```python
from build123d import *

# Parameters (mm, degrees)
SKETCH1_W           = 6
SKETCH1_H           = 6
BOSS_EXTRUDE1_DEPTH = 5
CUT_EXTRUDE1_DEPTH  = 1
CUT_EXTRUDE2_DEPTH  = 2
CUT_EXTRUDE3_DEPTH  = 2


with BuildPart() as part:
    # Sketch1 → Boss-Extrude1 (new body)
    with BuildSketch(Plane(origin=(0, 0, 0), x_dir=(1, 0, 0), z_dir=(0, 1, 0))):
        Rectangle(SKETCH1_W, SKETCH1_H)
    extrude(amount=BOSS_EXTRUDE1_DEPTH)

    # Sketch2 → Cut-Extrude1 (cut, symmetric)
    with BuildSketch(Plane(origin=(0, 0, 0), x_dir=(0, 0, -1), z_dir=(1, 0, 0))):
        Polygon((-3, 0), (3, 0), (3, 1), align=None)
        Polygon((3, 5), (-3, 5), (-3, 3), align=None)
    extrude(amount=CUT_EXTRUDE1_DEPTH, both=True, mode=Mode.SUBTRACT)

    # Sketch3 → Cut-Extrude2 (cut)
    with BuildSketch(Plane.ZY.offset(3)):
        Polygon((-3, 4), (3, 2), (3, 5), (-3, 5), align=None)
    extrude(amount=-CUT_EXTRUDE2_DEPTH, mode=Mode.SUBTRACT)

    # Sketch4 → Cut-Extrude3 (cut)
    with BuildSketch(Plane.ZY.offset(-1)):
        Polygon((3, 5), (-3, 5), (3, 4), align=None)
    extrude(amount=-CUT_EXTRUDE3_DEPTH, mode=Mode.SUBTRACT)


solid = part.part
```
The listing builds one solid part. Answer for the finished solid, in the listing's coordinates (mm). A direction names the side the tool comes from. Coordinates: 2 decimals unless noted, no trailing zeros. Loops run counter-clockwise (first coordinate to the right, second up) from the corner with the lowest first, then second, coordinate; pieces in that order, holes last. Notation, with made-up numbers: (62, 31.5) -> (66, 31.5) arc R11 ccw to (66, 39.5) -> close; hole circle Ø10 at (-27.75, 29.25). An arc over 180 degrees is marked (long way). Return JSON: item names as keys, results as strings. Group by question number.
(1) A cutting plane is placed at D-D on y = 2.55. Write down the section's boundary in (x, z), and give its area (3 significant figures).
(2) A cutting plane is placed at C-C on x = 1.85. Write down the section's boundary in (y, z).
(3) A cutting plane is placed at B-B on z = 2. Write down the section's boundary in (x, y).
(4) A cutting plane is placed at A-A on y = 3.55. Write down the section's boundary in (x, z), and give its area (3 significant figures).
(5) Which of the six approach directions +Z, -Z, +X, -X, +Y, -Y give full straight-line access (tool end or side, diameter ignored) to faces 1 (the flat face through (-2, 0, 0)), 2 (the flat face through (-1, 0.3, -1.3)), 3 (the flat face through (-1, 3.6, 0))?
(6) Find the intervals of material crossed by probe 1 along X at (y, z) = (3.65, -1.25); probe 2 along X at (y, z) = (0.55, -1.5); probe 3 along Y at (x, z) = (-1.65, 2.5), in increasing order. Write a range as from..to.
(7) Given pin 1 Ø1.5 at (y, z) = (4, -0.5) entering from -X; pin 2 Ø3 at (x, z) = (1, 1.5) entering from +Y, each flat-ended and moving along its own axis, determine where each tip first touches the part or whether it passes through.
The answers:
{
 "1": {"outline": "(-3, -3) -> (3, -3) -> (3, 3) -> (-1, 3) -> (-1, 1.35) -> (-3, 1.35) -> close", "area": "32.7 mm^2"},
 "2": {"outline": "(0, -3) -> (5, -3) -> (4, 3) -> (0, 3) -> close"},
 "3": {"outline": "(-3, 0) -> (-1, 0) -> (-1, 0.17) -> (1, 0.17) -> (1, 0) -> (3, 0) -> (3, 4.17) -> (1, 4.17) -> (1, 3.33) -> (-1, 3.33) -> (-1, 2.33) -> (-3, 2.33) -> close"},
 "4": {"outline": "(-3, -3) -> (3, -3) -> (3, 3) -> (1, 3) -> (1, 1.35) -> (-1, 1.35) -> (-1, -1.65) -> (-3, -1.65) -> close", "area": "23.4 mm^2"},
 "5": {"face 1": "+Z, -Z, +X, -X, -Y", "face 2": "-Z, -Y", "face 3": "+Z, -X, +Y"},
 "6": {"probe 1": "x = -1..3", "probe 2": "x = -3..-1, 1..3", "probe 3": "y = 0..2.17"},
 "7": {"pin 1": "stops at x = -1", "pin 2": "stops at y = 4.5"}
}
